from build123d import *

# Parameters (mm, degrees)
SKETCH2_W                  = 20
SKETCH2_H                  = 20
BOSS_EXTRUDE1_DEPTH        = 7.5
SKETCH3_W                  = 20
SKETCH3_H                  = 3
CUT_EXTRUDE1_DEPTH         = 10
SKETCH4_W                  = 7
SKETCH4_H                  = 7
CUT_EXTRUDE2_DEPTH         = 2.6
SKETCH5_R                  = 2.1
CUT_EXTRUDE3_DEPTH         = 20.52562419
F_3_1_3_1_DIAMETER_HOLE1_D = 3.2
F_3_1_3_1_DIAMETER_HOLE2_D = 3.2


with BuildPart() as part:
    # Sketch2 → Boss-Extrude1 (new body)
    with BuildSketch(Plane(origin=(0, 0, 0), x_dir=(1, 0, 0), z_dir=(0, 1, 0))):
        Rectangle(SKETCH2_W, SKETCH2_H)
    extrude(amount=-BOSS_EXTRUDE1_DEPTH)

    # Sketch3 → Cut-Extrude1 (cut)
    with BuildSketch(Plane.XY.offset(10)):
        Rectangle(SKETCH3_W, SKETCH3_H)
    extrude(amount=-CUT_EXTRUDE1_DEPTH, mode=Mode.SUBTRACT)

    # Sketch4 → Cut-Extrude2 (cut)
    with BuildSketch(Plane.XY.offset(-5)):
        Rectangle(SKETCH4_W, SKETCH4_H)
    extrude(amount=-CUT_EXTRUDE2_DEPTH, mode=Mode.SUBTRACT)

    # Sketch5 → Cut-Extrude3 (cut, through all)
    with BuildSketch(Plane.XY.offset(-5)):
        Circle(SKETCH5_R)
    extrude(amount=-CUT_EXTRUDE3_DEPTH, mode=Mode.SUBTRACT)

    # Ø3.1 (3.1) Diameter Hole1 (through all)
    with Locations(Plane(origin=(0, -1.5, 0), x_dir=(1, 0, 0), z_dir=(0, 1, 0))):
        with Locations((-6, -5), (6, -5)):
            Hole(F_3_1_3_1_DIAMETER_HOLE1_D / 2)

    # Ø3.1 (3.1) Diameter Hole2 (through all)
    with Locations(Plane(origin=(0, 0, 0), x_dir=(1, 0, 0), z_dir=(0, 1, 0))):
        with Locations((-6, 5), (6, 5)):
            Hole(F_3_1_3_1_DIAMETER_HOLE2_D / 2)


solid = part.part
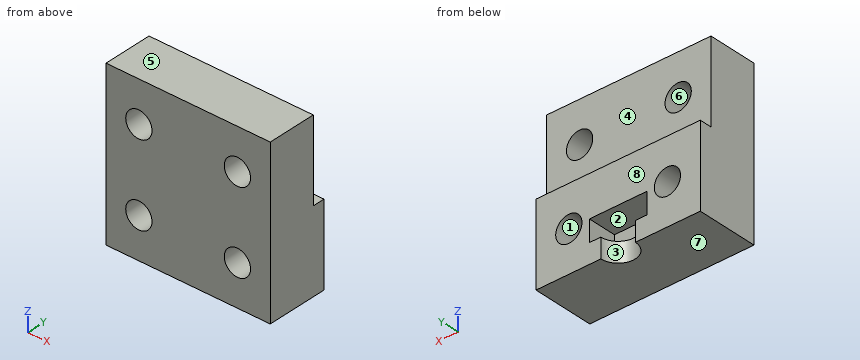
Geometry: final body of the model. Coordinates: model frame, mm. Face numbers are marked on the shaded views. A direction names the side the tool comes from. Give positions to 0.01 mm unless a question says otherwise; leave off trailing zeros. Loops run counter-clockwise (first coordinate to the right, second up) from the corner with the lowest first, then second, coordinate; pieces in that order, holes last. Notation, with made-up numbers: M 72.25,-22.5 L 81.25,-22.5 A28 ccw 81.25,9.5 Z; hole C 3,-10.75 d6. An arc over 180 degrees is marked long. Put each result on its own line as item: value.
1) Cut plane C-C, the plane x = 6. Return the cut outline in (y, z), plus the area to 3 significant figures.
Computed values:
outline: M -7.5,-10 L 0,-10 L 0,-6.6 L -7.5,-6.6 Z; M -7.5,-3.4 L 0,-3.4 L 0,0 L -1.5,0 L -1.5,3.4 L -7.5,3.4 Z; M -7.5,6.6 L -1.5,6.6 L -1.5,10 L -7.5,10 Z
area: 91.8 mm^2
2) Reachability of the marked faces 1, 2, 3, 4 and 5 from +Z, -Z, +X, -X, +Y, -Y: full face, straight path, thin tool, end or side. Return the list, or none.
Computed values:
face 1: +Y, -Y
face 2: +Y
face 3: -Z, +Y
face 4: +Z, +X, -X, +Y
face 5: +Z, +X, -X, +Y, -Y
3) Cut plane B-B, the plane y = -5.75. Return the cut outline in (x, z).
Computed values:
outline: M -10,-10 L 10,-10 L 10,10 L -10,10 Z; hole C -6,-5 d3.2; hole C -6,5 d3.2; hole C 6,-5 d3.2; hole C 6,5 d3.2
4) Cut plane A-A, the plane z = -4. Return the cut outline in (x, y).
Computed values:
outline: M -10,-7.5 L -7.25,-7.5 L -7.25,0 L -10,0 Z; M -4.75,-7.5 L 4.75,-7.5 L 4.75,0 L -4.75,0 Z; M 7.25,-7.5 L 10,-7.5 L 10,0 L 7.25,0 Z
5) First-contact query: P1, Ø1.9, axis at x = 6, z = 5, coming from the +Y side; P2, Ø6, axis at x = -1, z = 6.5, coming from the +Y side; P3, Ø0.8, axis at x = 4, y = -1, coming from the +Z side. Flat tips, straight axial feed; report the tip coordinate or a pass-through.
Computed values:
P1: passes through
P2: stops at y = -1.5
P3: stops at z = 0
6) Cut plane D-D, the plane x = -2.5. Return the cut outline in (y, z), plus the area to 3 significant figures.
Computed values:
outline: M -7.5,-10 L 0,-10 L 0,-7.6 L -3.5,-7.6 L -3.5,-5 L 0,-5 L 0,0 L -1.5,0 L -1.5,10 L -7.5,10 Z
area: 126 mm^2
7) Mould query, pull axis Z, two halves, no side actions, for the marked faces 6, 7 and 8. Classes: released by +Z, released by -Z, zero draft, split by the parting line, or undercut.
Computed values:
face 6: undercut
face 7: released by -Z
face 8: zero draft
8) Material intervals for L1, parallel to Z at x = 6, y = -3.35; L2, parallel to X at y = -3.7, z = 5; L3, parallel to Z at x = -3, y = -2.5, sorted ascending. Write a range as from..to.
Computed values:
L1: z = -10..-6.6, -3.4..3.4, 6.6..10
L2: x = -10..-7.6, -4.4..4.4, 7.6..10
L3: z = -10..-7.6, -5..10
